```python
from build123d import *


with BuildPart() as part:
    # Эскиз1 → Повернуть1 (revolve)
    with BuildSketch(Plane(origin=(0, 0, 0), x_dir=(1, 0, 0), z_dir=(0, 1, 0)), mode=Mode.PRIVATE) as revolve_1_sk:
        Polygon((0, 0), (12.7, 0), (12.7, -3), (15, -3), (15, -4), (29, -4), (29.8, -4.8), (29.8, -16), (32.25, -18.45), (32.25, -33.45), (31.5, -34.2), (31.5, -48.72), (30.5, -49.72), (26.8, -49.72), (25.8, -50.72), (25.8, -85.17), (24.8, -86.17), (0, -86.17), align=None)
    revolve(revolve_1_sk.sketch.rotate(Axis((0, 0, 0), (0, 0, 1)), 180), axis=Axis((0, 0, 0), (0, 0, 1)))

    # Эскиз2 → Повернуть2 (revolve)
    with BuildSketch(Plane(origin=(0, 0, 0), x_dir=(1, 0, 0), z_dir=(0, 1, 0))):
        with BuildLine():
            Line((0, -86.17), (0, -89.17))
            ThreePointArc((0, -89.17), (10.83404162, -88.416370928), (21.459399602, -86.17))
            Line((21.459399602, -86.17), (0, -86.17))
        make_face()
    revolve(axis=Axis((0, 0, 2.482382031), (0, 0, -1)))


solid = part.part
```
CAD build for the part. Positions are in the model's coordinates, mm. A direction names the side the tool comes from. Round coordinates to 2 decimals unless told otherwise and drop trailing zeros. Loops run counter-clockwise (first coordinate to the right, second up) from the corner with the lowest first, then second, coordinate; pieces in that order, holes last. Notation, with made-up numbers: M 41,7.25 L 81,7.25 A27 ccw 81,43.25 Z; hole C 38.25,61.5 d2. An arc over 180 degrees is marked long. Use a Markdown table: item, result. Add a question column.
(1) Flat gauge pins, fed straight in: pin 1 (3 mm diameter, centred on x = 16, y = 13, fed in from +Z); pin 2 (3 mm diameter, centred on x = -5.5, y = -3.5, fed in from +Z); pin 3 (2 mm diameter, centred on x = -17, z = 39.5, fed in from -Y); pin 4 (4 mm diameter, centred on x = -3, y = 2, fed in from -Z). Where does each tip first touch, or does it go through?
(2) Drill centre lines: line 1 (X direction, y = -0.5, z = 15); line 2 (Z direction, x = -4, y = -24); line 3 (Z direction, x = -1, y = 27). Where is each one in solid material? Low to high.
(3) Cut at D-D (z = 41). Give the cut face in (x, y), and give its area (3 significant figures).
(4) Cut at C-C (z = 68). Give the cut face in (x, y).
(5) Which spindle directions (+Z, -Z, +X, -X, +Y, -Y) get a long thin tool onto all of the face, cutting with end or side? Do faces 1 (the face through (0, 0, 0)), 2 (the face through (-8.06, -12.65, 3.51)), 3 (the face through (0, 27, 49.72)). Say none if no direction does.
Geometry says:
| question | item | result |
|---|---|---|
| 1 | pin 1 | stops at z = 86.8 |
| 1 | pin 2 | stops at z = 89.01 |
| 1 | pin 3 | stops at y = -27.13 |
| 1 | pin 4 | stops at z = 0 |
| 2 | line 1 | x = -29.8 to 29.8 |
| 2 | line 2 | z = 4 to 86.17 |
| 2 | line 3 | z = 4 to 49.72 |
| 3 | outline | C 0,0 d63 |
| 3 | area | 3,120 mm² |
| 4 | outline | C 0,0 d51.6 |
| 5 | face 1 | -Z, +X, -X, +Y, -Y |
| 5 | face 2 | -Z |
| 5 | face 3 | +Z |
